Design review of the part built by this model. Coordinates are the model's own, in mm. Face numbers are marked on the shaded views. A direction names the side the tool comes from. Give positions to 0.01 mm unless a question says otherwise; leave off trailing zeros. Write each loop counter-clockwise with the first axis right and the second up, starting at its lowest first coordinate (ties: lowest second). Pieces come first, ordered by that corner, then holes. Notation, with made-up numbers: M 18.5,-29 L 72.5,-29 A16 cw 72.5,-20 Z; hole C 76,7 d2. An arc over 180 degrees is marked long. Answer in a Markdown table with one row per item.
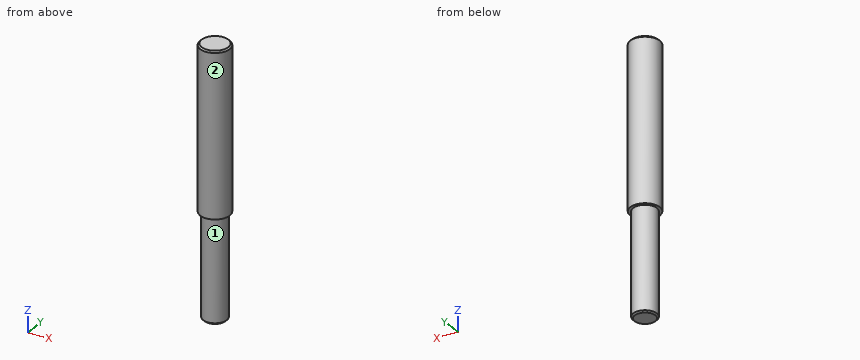
```python
from build123d import *

# Parameters (mm, degrees)
SKETCH1_R           = 1
BOSS_EXTRUDE1_DEPTH = 18
SKETCH2_OUTSIDE_W   = 7.644
SKETCH2_OUTSIDE_H   = 7.644
SKETCH2_OUTSIDE_R   = 0.8
CUT_EXTRUDE1_DEPTH  = 7
CHAMFER1_SIZE       = 0.1
CHAMFER2_SIZE       = 0.1


with BuildPart() as part:
    # Sketch1 → Boss-Extrude1 (new body)
    with BuildSketch(Plane.XY):
        Circle(SKETCH1_R)
    extrude(amount=-BOSS_EXTRUDE1_DEPTH)

    # Sketch2 outside → Cut-Extrude1 (cut)
    with BuildSketch(Plane(origin=(0, 0, -18), x_dir=(-1, 0, 0), z_dir=(0, 0, -1))):
        Rectangle(SKETCH2_OUTSIDE_W, SKETCH2_OUTSIDE_H)
        Circle(SKETCH2_OUTSIDE_R, mode=Mode.SUBTRACT)
    extrude(amount=-CUT_EXTRUDE1_DEPTH, mode=Mode.SUBTRACT)

    # Chamfer1
    chamfer1_edges = [part.edges().sort_by_distance(p)[0] for p in [
        (0.8, 0, -18),
    ]]
    chamfer(chamfer1_edges, length=CHAMFER1_SIZE)

    # Chamfer2
    chamfer2_edges = [part.edges().sort_by_distance(p)[0] for p in [
        (-1, 0, 0),
    ]]
    chamfer(chamfer2_edges, length=CHAMFER2_SIZE)


solid = part.part
```
1) Add section C-C (z = -6.5). Write out the cut boundary in (x, y).
Geometry says:
| item | result |
|---|---|
| outline | C 0,0 d2 |
2) For the marked faces 1 and 2, list the 3-axis set-ups (+Z, -Z, +X, -X, +Y, -Y) from which the entire face can be reached by the end or side of a thin tool; tool diameter is ignored.
Geometry says:
| item | result |
|---|---|
| face 1 | -Z |
| face 2 | +Z, -Z |
3) Add section A-A (y = 0). Write out the cut boundary in (x, z), and give its area (3 significant figures).
Geometry says:
| item | result |
|---|---|
| outline | M -1,-11 L -0.8,-11 L -0.8,-17.9 L -0.7,-18 L 0.7,-18 L 0.8,-17.9 L 0.8,-11 L 1,-11 L 1,-0.1 L 0.9,0 L -0.9,0 L -1,-0.1 Z |
| area | 33.2 mm^2 |
4) To check wall thickness, follow probe 1 along Y at (x, z) = (0.6, -7.25); probe 2 along Z at (x, y) = (0.8, 0.3). State the ranges of each line that lie inside material, in increasing order. Write a range as [from, to].
Geometry says:
| item | result |
|---|---|
| probe 1 | [-0.8, 0.8] |
| probe 2 | [-11, 0] |
